from build123d import *

# Parameters (mm, degrees)
F1_DEPTH = 12.7
F2_D     = 3.7973
F2_DEPTH = 15.8877
F2_TIP   = 1.1408240143
F3_D     = 16.66748
F3_DEPTH = 15.9004
F3_TIP   = 5.0074161752
F4_D     = 7.9375
F4_DEPTH = 17.4879
F4_TIP   = 2.3846655818
F5_D     = 10.0838
F5_DEPTH = 17.5006
F5_TIP   = 3.0294791551
F6_D     = 7.9375
F6_DEPTH = 20.6756
F6_TIP   = 2.3846655818


with BuildPart() as f1:
    # F0 (on Front) → F1 (new body)
    with BuildSketch(Plane.XZ):
        Polygon((-304.8, 0), (0, 0), (0, 95.2246), (-12.7254, 95.2246), (-12.7254, 133.3754), (0, 133.3754), (0, 273.0246), (-12.7254, 273.0246), (-12.7254, 311.1754), (0, 311.1754), (0, 406.4), (-304.8, 406.4), (-304.8, 311.1754), (-292.0746, 311.1754), (-292.0746, 273.0246), (-304.8, 273.0246), (-304.8, 133.3754), (-292.0746, 133.3754), (-292.0746, 95.2246), (-304.8, 95.2246), align=None)
    extrude(amount=F1_DEPTH)

    # F2
    with Locations(Plane(origin=(0, 0, 0), x_dir=(1, 0, 0), z_dir=(0, 1, 0))):
        with Locations((-276.225, -374.65), (-276.225, -260.35), (-276.225, -146.05), (-276.225, -31.75), (-28.575, -374.65), (-28.575, -260.35), (-28.575, -146.05), (-28.575, -31.75)):
            Hole(F2_D / 2, depth=F2_DEPTH)
            with Locations((0, 0, -(F2_DEPTH + F2_TIP / 2))):  # 118° drill point
                Cone(0, F2_D / 2, F2_TIP, mode=Mode.SUBTRACT)

    # F3
    with Locations(Plane(origin=(0, 0, 0), x_dir=(1, 0, 0), z_dir=(0, 1, 0))):
        with Locations((-152.4, -203.2)):
            Hole(F3_D / 2, depth=F3_DEPTH)
            with Locations((0, 0, -(F3_DEPTH + F3_TIP / 2))):  # 118° drill point
                Cone(0, F3_D / 2, F3_TIP, mode=Mode.SUBTRACT)

    # F4
    with Locations(Plane(origin=(0, 0, 0), x_dir=(1, 0, 0), z_dir=(0, 1, 0))):
        with Locations((-263.525, -381), (-263.525, -203.2), (-263.525, -25.4), (-41.275, -381), (-41.275, -203.2), (-41.275, -25.4)):
            Hole(F4_D / 2, depth=F4_DEPTH)
            with Locations((0, 0, -(F4_DEPTH + F4_TIP / 2))):  # 118° drill point
                Cone(0, F4_D / 2, F4_TIP, mode=Mode.SUBTRACT)

    # F5
    with Locations(Plane(origin=(0, 0, 0), x_dir=(1, 0, 0), z_dir=(0, 1, 0))):
        with Locations((-231.775, -381), (-231.775, -203.2), (-231.775, -25.4), (-73.025, -25.4), (-73.025, -203.2), (-73.025, -381)):
            Hole(F5_D / 2, depth=F5_DEPTH)
            with Locations((0, 0, -(F5_DEPTH + F5_TIP / 2))):  # 118° drill point
                Cone(0, F5_D / 2, F5_TIP, mode=Mode.SUBTRACT)

    # F6
    with Locations(Plane(origin=(0, 0, 0), x_dir=(1, 0, 0), z_dir=(0, 1, 0))):
        with Locations((-225.425, -96.8375), (-79.375, -96.8375)):
            Hole(F6_D / 2, depth=F6_DEPTH)
            with Locations((0, 0, -(F6_DEPTH + F6_TIP / 2))):  # 118° drill point
                Cone(0, F6_D / 2, F6_TIP, mode=Mode.SUBTRACT)


solid = f1.part
Geometry: final body of the model. Coordinates: model frame, mm. A direction names the side the tool comes from. Give positions to 0.01 mm unless a question says otherwise; leave off trailing zeros. Put each result on its own line as item: value.
Q1. Draft query along X for faces 1 (the face through (-299, -6, 311.175)), 2 (the face through (0, -6, 202)), 3 (the face through (-72.37, -6.44, 20.4)). Return one class per face: released by +X, released by -X, zero draft, split by the parting line, or undercut.
Here are the results:
face 1: zero draft
face 2: released by +X
face 3: undercut
Q2. Pin query (flat end, axial travel): pin 1 (6.5 mm diameter, centred on x = -263.525, z = 381, fed in from +Y); pin 2 (6 mm diameter, centred on y = -7, z = 300.5, fed in from -X). Return the tip coordinate at first contact, or that it passes through.
Here are the results:
pin 1: passes through
pin 2: stops at x = -292.07
Q3. Material intervals for L1, parallel to X at y = -6.75, z = 260.35; L2, parallel to X at y = -3.75, z = 203.2; L3, parallel to Z at x = -72.5, y = -6.25, sorted ascending.
Here are the results:
L1: x = -304.8 to -278.12, -274.33 to -30.47, -26.68 to 0
L2: x = -304.8 to -267.49, -259.56 to -236.82, -226.73 to -160.73, -144.07 to -78.07, -67.98 to -45.24, -37.31 to 0
L3: z = 0 to 20.39, 30.41 to 198.19, 208.21 to 375.99, 386.01 to 406.4
Q4. Section A-A, the plane y = -10.25. Count the separate pieces of the cut face and the enclosed holes in it, then the cut area to 3 significant figures.
Here are the results:
separate pieces: 1
enclosed holes: 23
area: 121,000 mm^2
Q5. Reachability of faces 4 (the face through (-267.31, -6.44, 24.21)), 5 (the face through (-12.725, -6, 292)), 6 (the face through (-299, -6, 133.375)) from +Z, -Z, +X, -X, +Y, -Y: full face, straight path, thin tool, end or side. Return the list, or none.
Here are the results:
face 4: +Y, -Y
face 5: +X, +Y, -Y
face 6: -X, +Y, -Y
